```python
from build123d import *

# Parameters (mm, degrees)
SKETCH3_W           = 3.6
SKETCH3_H           = 3.6
CUT_EXTRUDE2_DEPTH  = 3.5
SKETCH4_W           = 4.2
SKETCH4_H           = 5
BOSS_EXTRUDE1_DEPTH = 2.61
FILLET1_R           = 1


with BuildPart() as part:
    # Sketch1 → Revolve1 (revolve)
    with BuildSketch(Plane.XY, mode=Mode.PRIVATE) as revolve1_sk:
        Polygon((0, 0), (0, 10), (4, 10), (3.5, 8), (3.5, 0), align=None)
    revolve(revolve1_sk.sketch.rotate(Axis((0, 0, 0), (0, 1, 0)), 90), axis=Axis((0, 0, 0), (0, 1, 0)))

    # Sketch3 → Cut-Extrude2 (cut)
    with BuildSketch(Plane.XZ):
        Rectangle(SKETCH3_W, SKETCH3_H)
    extrude(amount=-CUT_EXTRUDE2_DEPTH, mode=Mode.SUBTRACT)

    # Sketch4 → Boss-Extrude1 (add)
    with BuildSketch(Plane(origin=(0, 0, 0), x_dir=(1, 0, 0), z_dir=(0, 1, 0))):
        with Locations((-3.9, 0)):
            Rectangle(SKETCH4_W, SKETCH4_H)
        with Locations((3.9, 0)):
            Rectangle(SKETCH4_W, SKETCH4_H)
    extrude(amount=BOSS_EXTRUDE1_DEPTH)

    # Fillet1
    fillet1_edges = [part.edges().sort_by_distance(p)[0] for p in [
        (-2.449489743, 1.305, -2.5),
        (-2.449489743, 1.305, 2.5),
        (-6, 1.305, -2.5),
        (-6, 1.305, 2.5),
        (0, 10, 4),
        (2.449489743, 1.305, 2.5),
        (2.449489743, 1.305, -2.5),
        (6, 1.305, 2.5),
        (6, 1.305, -2.5),
    ]]
    fillet(fillet1_edges, radius=FILLET1_R)


solid = part.part
```
Verification items for the finished model (mm, model axes). A direction names the side the tool comes from. Give positions to 0.01 mm unless a question says otherwise; leave off trailing zeros. Loops run counter-clockwise (first coordinate to the right, second up) from the corner with the lowest first, then second, coordinate; pieces in that order, holes last. Notation, with made-up numbers: M 81.5,47 L 139.5,47 A25 ccw 139.5,78 Z; hole C 14,-21.5 d11. An arc over 180 degrees is marked long. One line per question, with ' | ' between items.
Item 1: Section check C-C, the plane z = 0. Record the cut outline in (x, y), plus the area to 3 significant figures.
Completed:
outline: M -6,0 L -1.8,0 L -1.8,3.5 L 1.8,3.5 L 1.8,0 L 6,0 L 6,2.61 L 3.5,2.61 L 3.5,8 L 3.69,8.76 A1 ccw 2.72,10 L -2.72,10 A1 ccw -3.69,8.76 L -3.5,8 L -3.5,2.61 L -6,2.61 Z | area: 70.7 mm^2
Item 2: Section check A-A, the plane y = 1.75. Record the cut outline in (x, z).
Completed:
outline: M -6,-1.5 A1 ccw -5,-2.5 L -2.83,-2.5 A1 cw -2.2,-2.72 A3.5 ccw 2.2,-2.72 A1 cw 2.83,-2.5 L 5,-2.5 A1 ccw 6,-1.5 L 6,1.5 A1 ccw 5,2.5 L 2.83,2.5 A1 cw 2.2,2.72 A3.5 ccw -2.2,2.72 A1 cw -2.83,2.5 L -5,2.5 A1 ccw -6,1.5 Z; hole M -1.8,-1.8 L 1.8,-1.8 L 1.8,1.8 L -1.8,1.8 Z
Item 3: Section check B-B, the plane x = 0. Record the cut outline in (y, z).
Completed:
outline: M 0,-3.5 L 8,-3.5 L 8.76,-3.69 A1 ccw 10,-2.72 L 10,2.72 A1 ccw 8.76,3.69 L 8,3.5 L 0,3.5 L 0,1.8 L 3.5,1.8 L 3.5,-1.8 L 0,-1.8 Z
Item 4: Draft check along Z on faces 5 (the face through (-1.8, 2, 0)), 6 (the face through (0, 10, 0)), 7 (the face through (5.715, 1.323, 2.199)). Enter one of: +Z half, -Z half, draft (parallel to the pull), parting line (faces both ways), or undercut.
Completed:
face 5: undercut | face 6: draft | face 7: +Z half
Item 5: Tool access check on faces 1 (the face through (3.105, 4.833, -1.615)), 2 (the face through (4, 1, -2.5)), 3 (the face through (1.8, 2, 0)), 4 (the face through (4, 1, 2.5)). Record the directions out of +Z, -Z, +X, -X, +Y, -Y that give a thin tool (end or side, any length) a straight path to the whole face; none if there is none.
Completed:
face 1: none | face 2: -Z, +X, +Y, -Y | face 3: -Y | face 4: +Z, +X, +Y, -Y
Item 6: Thickness scan on line 1 (X direction, y = 1.75, z = -1.5); line 2 (Y direction, x = -4, z = -1); line 3 (Z direction, x = -3.25, y = 2.25). Record the ranges inside material, lowest first. Write a range as [from, to].
Completed:
line 1: x = [-6, -1.8], [1.8, 6] | line 2: y = [0, 2.61] | line 3: z = [-2.5, 2.5]
Item 7: Section check D-D, the plane y = 4.25. Record the cut outline in (x, z), plus the area to 3 significant figures.
Completed:
outline: C 0,0 d7 | area: 38.5 mm^2
Item 8: Depth check by flat-ended pin: P1, Ø3, axis at x = 0, y = 1, coming from the -Z side; P2, Ø1.1, axis at x = 4, y = 1.5, coming from the -Z side; P3, Ø3, axis at x = 0.5, y = 2.5, coming from the +Z side. Enter the tip coordinate at first touch or a pass-through.
Completed:
P1: stops at z = -3.5 | P2: stops at z = -2.5 | P3: stops at z = 3.5
